Here's the drawing with two shaded views (mm, measured from the low corner). I have some questions. Coordinates: 2 decimals unless noted, no trailing zeros. Write each loop counter-clockwise with the first axis right and the second up, starting at its lowest first coordinate (ties: lowest second). Pieces come first, ordered by that corner, then holes. Notation, with made-up numbers: (81, 87.5) -> (140, 87.5) arc R7 cw to (140, 95.5) -> close; hole circle Ø8 at (49, 83.25). An arc over 180 degrees is marked (long way). Use one line per item in the form item = value.
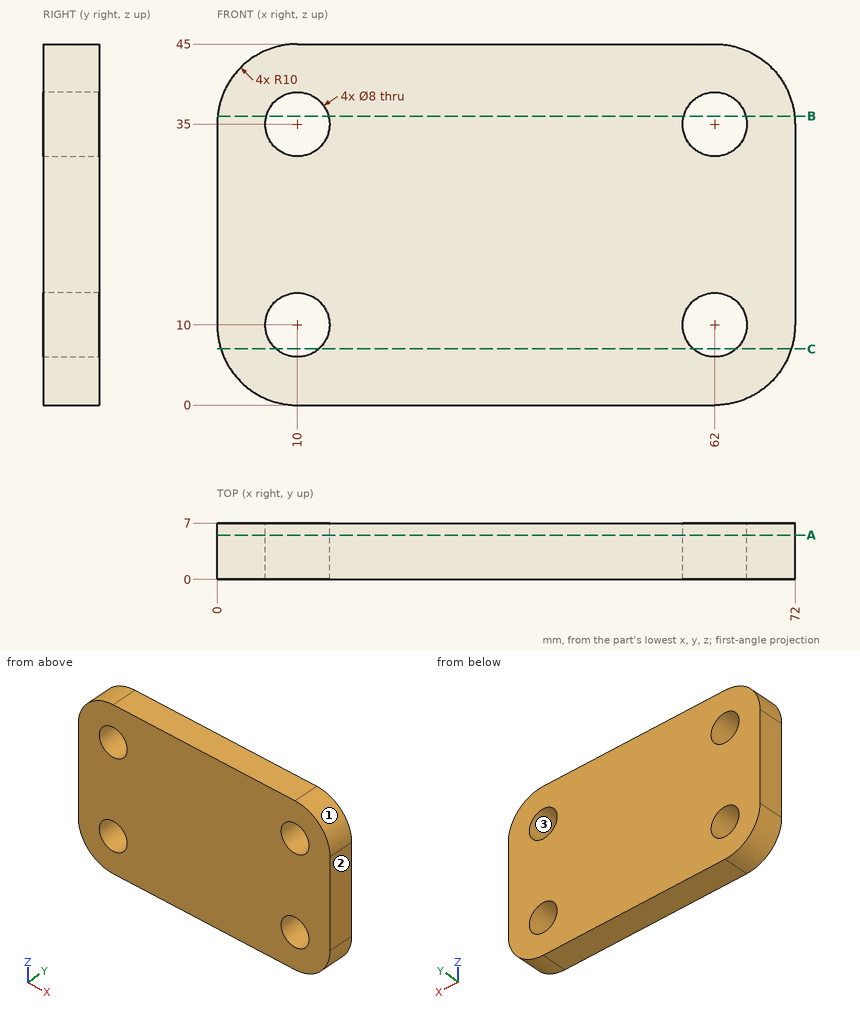
Q1. Suppose I cut it at C-C (z = 7). Write out the boundary of the cut face in (x, y).
Return value:
outline = (0.46, 0) -> (7.35, 0) -> (7.35, 7) -> (0.46, 7) -> close; (12.65, 0) -> (59.35, 0) -> (59.35, 7) -> (12.65, 7) -> close; (64.65, 0) -> (71.54, 0) -> (71.54, 7) -> (64.65, 7) -> close
Q2. Suppose I cut it at A-A (y = 5.5). Write out the boundary of the cut face in (x, z), then the cut area to 3 significant figures.
Return value:
outline = (0, 10) arc R10 ccw to (10, 0) -> (62, 0) arc R10 ccw to (72, 10) -> (72, 35) arc R10 ccw to (62, 45) -> (10, 45) arc R10 ccw to (0, 35) -> close; hole circle Ø8 at (10, 10); hole circle Ø8 at (10, 35); hole circle Ø8 at (62, 10); hole circle Ø8 at (62, 35)
area = 2,950 mm2
Q3. Thinking about a two-plate mould opening in Z: for the marked faces 1, 2 and 3, which applies, released by +Z, released by -Z, zero draft, split by the parting line, or undercut?
Return value:
face_1 = released by +Z
face_2 = zero draft
face_3 = undercut
Q4. Suppose I cut it at B-B (z = 36). Write out the boundary of the cut face in (x, y).
Return value:
outline = (0.05, 0) -> (6.13, 0) -> (6.13, 7) -> (0.05, 7) -> close; (13.87, 0) -> (58.13, 0) -> (58.13, 7) -> (13.87, 7) -> close; (65.87, 0) -> (71.95, 0) -> (71.95, 7) -> (65.87, 7) -> close
Q5. Will this pin go through, and if not, where does the flat tip stop? pin 1 (4 mm diameter, centred on y = 3, z = 5.5, fed in from -X).
Return value:
pin_1 = 0.32
Q6. If I drill on line 1 (X direction, y = 2.5, z = 10); line 2 (Z direction, x = 10.5, y = 4); line 3 (Z direction, x = 65, y = 4.5), over which ranges is the centre line in solid material (lowest first)? Write a range as from..to.
Return value:
line_1 = 0..6, 14..58, 66..72
line_2 = 0..6.03, 13.97..31.03, 38.97..45
line_3 = 0.46..7.35, 12.65..32.35, 37.65..44.54
